from build123d import *

# Parameters (mm, degrees)
SKETCH2_R          = 2.1
BASE_FLANGE1_DEPTH = 0.5
FILLET1_R          = 3.5
FILLET2_R          = 0.9


# Sheet-metal steps are written as plain solids
with BuildPart() as part:
    # Base-Flange1: sheet metal written as solids
    # Sketch2 → Base-Flange1 (new body)
    with BuildSketch(Plane(origin=(0, 0, 0), x_dir=(1, 0, 0), z_dir=(0, 1, 0))):
        Polygon((-9.5, 0), (9.5, 0), (9.5, -10), (23.5, -10), (23.5, 7), (4.5, 7), (4.5, 10), (24.5, 10), (24.5, 11.9), (4.5, 11.9), (4.5, 17.9), (-4.5, 17.9), (-4.5, 11.9), (-24.5, 11.9), (-24.5, 10), (-4.5, 10), (-4.5, 7), (-23.5, 7), (-23.5, -10), (-9.5, -10), align=None)
        with Locations(Location((16.5, -4, 0), (0, 0, 270))):
            Circle(SKETCH2_R, mode=Mode.SUBTRACT)
        with Locations(Location((-16.5, -4, 0), (0, 0, 90))):
            Circle(SKETCH2_R, mode=Mode.SUBTRACT)
    extrude(amount=-BASE_FLANGE1_DEPTH)

    # Fillet1
    # the kernel refuses this fillet: 3.5 mm, written as the material it adds along each edge
    with BuildSketch(Plane(origin=(9.5, 0, 0), x_dir=(-1, 0, 0), z_dir=(0, -1, 0))) as fillet1_piece_1:
        with BuildLine():
            CenterArc((FILLET1_R, -FILLET1_R), FILLET1_R, 90, 90)
            Line((0, -FILLET1_R), (0, 0))
            Line((0, 0), (FILLET1_R, 0))
        make_face()
    extrude(amount=0.5)
    with BuildSketch(Plane(origin=(-9.5, 0, 0), x_dir=(1, 0, 0), z_dir=(0, -1, 0))) as fillet1_piece_2:
        with BuildLine():
            CenterArc((FILLET1_R, FILLET1_R), FILLET1_R, 180, 90)
            Line((0, FILLET1_R), (0, 0))
            Line((0, 0), (FILLET1_R, 0))
        make_face()
    extrude(amount=0.5)
    with BuildSketch(Plane(origin=(-4.5, 0, -7), x_dir=(0, 0, -1), z_dir=(0, -1, 0))) as fillet1_piece_3:
        with BuildLine():
            CenterArc((3.5, -3.464101615), FILLET1_R, 98.213210702, 81.786789298)
            Line((0, -3.464101615), (0, 0))
            Line((0, 0), (3, 0))
        make_face()
    extrude(amount=0.5)
    with BuildSketch(Plane(origin=(4.5, 0, -7), x_dir=(1, 0, 0), z_dir=(0, -1, 0))) as fillet1_piece_4:
        with BuildLine():
            CenterArc((3.464101615, -3.5), FILLET1_R, 90, 81.786789298)
            Line((0, -3), (0, 0))
            Line((0, 0), (3.464101615, 0))
        make_face()
    extrude(amount=0.5)
    # the kernel refuses this fillet: 3.5 mm, written as the material it takes off along each edge
    with BuildSketch(Plane(origin=(-9.5, 8.75, 10), x_dir=(-1, 0, 0), z_dir=(0, -1, 0)), Plane(origin=(-23.5, 8.75, 10), x_dir=(0, 0, -1), z_dir=(0, -1, 0)), Plane(origin=(-23.5, 8.75, -7), x_dir=(1, 0, 0), z_dir=(0, -1, 0)), Plane(origin=(-4.5, 8.75, -17.9), x_dir=(1, 0, 0), z_dir=(0, -1, 0)), Plane(origin=(4.5, 8.75, -17.9), x_dir=(0, 0, 1), z_dir=(0, -1, 0)), Plane(origin=(23.5, 8.75, -7), x_dir=(0, 0, 1), z_dir=(0, -1, 0)), Plane(origin=(23.5, 8.75, 10), x_dir=(-1, 0, 0), z_dir=(0, -1, 0)), Plane(origin=(9.5, 8.75, 10), x_dir=(0, 0, -1), z_dir=(0, -1, 0))) as fillet1_2_piece_1:
        with BuildLine():
            CenterArc((FILLET1_R, FILLET1_R), FILLET1_R, 180, 90)
            Line((0, FILLET1_R), (0, 0))
            Line((0, 0), (FILLET1_R, 0))
        make_face()
    extrude(amount=18, mode=Mode.SUBTRACT)

    # Fillet2
    fillet2_edges = [part.edges().sort_by_distance(p)[0] for p in [
        (-24.5, -0.25, -10),
        (-24.5, -0.25, -11.9),
        (24.5, -0.25, -11.9),
        (24.5, -0.25, -10),
    ]]
    fillet(fillet2_edges, radius=FILLET2_R)


solid = part.part
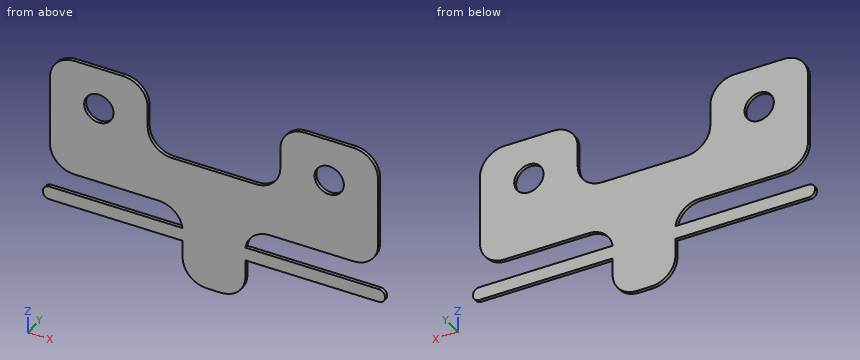
Model file for the job. Use its own axes, mm. Give positions to 0.01 mm unless a question says otherwise; leave off trailing zeros. Order: outer loops, then holes, each group sorted by start corner. A loop starts at its lowest first (then second) coordinate and runs counter-clockwise, first axis right, second up. Notation, with made-up numbers: (-12, 56.25) - (6, 56.25) arc R17 cw to (6, 70.25) - close; hole circle Ø4 at (36.25, 73). An arc over 180 degrees is marked (long way). Return JSON: item names as keys, results as strings.
1) Probe line 1 (X direction, y = -0.3, z = 4); line 2 (Z direction, x = -16.5, y = -0.4); line 3 (X direction, y = -0.15, z = -1). List the from-to ranges inside material, lowest first. Write a range as from..to.
Geometry says:
{"line 1": "-23.5..-18.6, -14.4..-9.5, 9.5..14.4, 18.6..23.5", "line 2": "-11.9..-10, -7..1.9, 6.1..10", "line 3": "-23.5..23.5"}
2) Cut at D-D, the plane x = -11. Give the cut face in (y, z).
Geometry says:
{"outline": "(-0.5, -11.9) - (0, -11.9) - (0, -10) - (-0.5, -10) - close; (-0.5, -7) - (0, -7) - (0, 9.37) - (-0.5, 9.37) - close"}
3) Cut at C-C, the plane z = 0.75. Give the cut face in (x, y).
Geometry says:
{"outline": "(-23.5, -0.5) - (-8.17, -0.5) - (-8.17, 0) - (-23.5, 0) - close; (8.17, -0.5) - (23.5, -0.5) - (23.5, 0) - (8.17, 0) - close"}
4) Flat gauge pin, fed straight in: P1, Ø4, axis at x = -16.5, z = 4, coming from the +Y side. Where does the tip first touch, or does it go through?
Geometry says:
{"P1": "through"}
5) Cut at A-A, the plane x = 16.5. Give the cut face in (y, z).
Geometry says:
{"outline": "(-0.5, -11.9) - (0, -11.9) - (0, -10) - (-0.5, -10) - close; (-0.5, -7) - (0, -7) - (0, 1.9) - (-0.5, 1.9) - close; (-0.5, 6.1) - (0, 6.1) - (0, 10) - (-0.5, 10) - close"}
6) Cut at B-B, the plane z = 4. Give the cut face in (x, y).
Geometry says:
{"outline": "(-23.5, -0.5) - (-18.6, -0.5) - (-18.6, 0) - (-23.5, 0) - close; (-14.4, -0.5) - (-9.5, -0.5) - (-9.5, 0) - (-14.4, 0) - close; (9.5, -0.5) - (14.4, -0.5) - (14.4, 0) - (9.5, 0) - close; (18.6, -0.5) - (23.5, -0.5) - (23.5, 0) - (18.6, 0) - close"}
